CAD build for the part. Positions are in the model's coordinates, mm. A direction names the side the tool comes from. Give positions to 0.01 mm unless a question says otherwise; leave off trailing zeros. Write each loop counter-clockwise with the first axis right and the second up, starting at its lowest first coordinate (ties: lowest second). Pieces come first, ordered by that corner, then holes. Notation, with made-up numbers: (-19.75, 24.5) -> (23.25, 24.5) arc R23 cw to (23.25, 59.5) -> close; hole circle Ø6 at (1.5, -19). An arc over 180 degrees is marked (long way). Answer as a JSON object with one key per item and string values.
Autodesk Inventor part; units mm, degrees
ref_plane "YZ Plane" through (0, 0, 0) normal (1, 0, 0) x (0, 1, 0)
ref_plane "XZ Plane" through (0, 0, 0) normal (0, 1, 0) x (-1, 0, 0)
ref_plane "XY Plane" through (0, 0, 0) normal (0, 0, 1) x (1, 0, 0)
sketch "Sketch1" plane through (0, 0, 0) normal (1, 0, 0) x (0, 1, 0)
  circle A0 centre (4.0001, 0) radius 1.25
  circle A1 centre (-3.9999, 0) radius 1.25
  circle A2 centre (0, 0) radius 11
  line L0 (11, 0) -> (11, -22)
  line L1 (11, 0) -> (33, 0) construction
  line L2 (-11, 0) -> (-11, -22)
  line L3 (-11, 0) -> (11, 0) construction
  circle A3 centre (0, -22) radius 11
  circle A4 centre (0, -26.0001) radius 1.25
  circle A5 centre (0, -18.0001) radius 1.25
  point P0 (1.5875, 1.5875)
  dimension "d0" = 22
  dimension "d1" = 90
  dimension "d2" = 22
  dimension "d3" = 90
extrude "Extrusion1" add sketch "Sketch1" along normal blind 5
sketch "Sketch2" plane through (5, 0, 0) normal (1, 0, 0) x (0, 0, -1)
  arc A0 (0, 11) -> (0, -11) centre (0, 0) ccw
  line L0 (0, -11) -> (22, -11)
  arc A1 (22, -11) -> (22, 11) centre (22, 0) ccw
  line L1 (22, 11) -> (0, 11)
  circle A2 centre (18.0001, 0) radius 1.25
  circle A3 centre (26.0001, 0) radius 1.25
  circle A4 centre (0, -3.9999) radius 1.25
  circle A5 centre (0, 4.0001) radius 1.25
extrude "Extrusion2" add sketch "Sketch2" along normal blind 3 and the other way blind 5 contours A4 | A5
sketch "Sketch3" plane through (0, 0, 0) normal (-1, 0, 0) x (0, 0, 1)
  arc A0 (0, -11) -> (0, 11) centre (0, 0) ccw
  line L0 (0, -11) -> (-22, -11)
  arc A1 (-22, 11) -> (-22, -11) centre (-22, 0) ccw
  line L1 (-22, 11) -> (0, 11)
  circle A2 centre (-18.0001, 0) radius 1.25
  circle A3 centre (-26.0001, 0) radius 1.25
  circle A4 centre (0, -3.9999) radius 1.25
  circle A5 centre (0, 4.0001) radius 1.25
extrude "Extrusion3" add sketch "Sketch3" against normal blind 5 contours A2 | A3
sketch "Sketch4" plane through (0, 0, 0) normal (-1, 0, 0) x (0, 0, 1)
  line L0 (0, 0) -> (-22, 0)
  line L1 (0, 0) -> (22, 0) construction
  circle A0 centre (-22, 0) radius 11
  circle A1 centre (-22, 0) radius 9.5
  dimension "d12" = 22
  dimension "d13" = 180
  dimension "d14" = 22
  dimension "d15" = 19
extrude "Extrusion4" add sketch "Sketch4" along normal blind 15 contours A1 | A0
sketch "Sketch5" plane through (5, 0, 0) normal (1, 0, 0) x (0, 0, -1)
  circle A0 centre (0, 0) radius 24.5
  circle A1 centre (-20, 0) radius 3.5
  circle A2 centre (-14.1421, 14.1421) radius 2.675
  circle A3 centre (-14.1421, -14.1421) radius 2.675
  circle A4 centre (14.1421, -14.1421) radius 2.675
  circle A5 centre (14.1421, 14.1421) radius 2.675
  circle A6 centre (0, 0) radius 11
  line L0 (0, -11) -> (22, -11)
  line L1 (22, 11) -> (0, 11)
  point P0 (0, 0)
  point P1 (21.8918, 11)
  point P2 (21.8918, -11)
extrude "Extrusion5" add sketch "Sketch5" along normal blind 5 contours A0 L0 A6 L1 picked at (19.9018, -1.2624)
sketch "Sketch6" plane through (-15, 0, -22) normal (-1, 0, 0) x (0, 0, 1)
  circle A0 centre (0, 0) radius 7.5
  point P0 (22, 0)
  dimension "d20" = 15
extrude "Extrusion6" cut sketch "Sketch6" against normal blind 15
properties part number "Herramienta Marcador Conector"
1) Mould opens along Y. For faces 1 (the cylindrical face through (-5, 0, -33)), 2 (the flat face through (8, 4, 0)), 3 (the cylindrical face through (6.48, 2.76, 0.16)), 4 (the flat face through (5, 11, -11)) say: released by +Y, released by -Y, zero draft, split by the parting line, or undercut.
Model answer:
{"face 1": "split by the parting line", "face 2": "undercut", "face 3": "undercut", "face 4": "released by +Y"}
2) Slice it at C-C (y = -9). List the corners of the cut face in (x, z), then the cut area to 3 significant figures.
Model answer:
{"outline": "(-15, -28.32) -> (5, -28.32) -> (5, -22.79) -> (10, -22.79) -> (10, -6.32) -> (5, -6.32) -> (5, 6.32) -> (0, 6.32) -> (0, -15.68) -> (-15, -15.68) -> close", "area": "445 mm2"}
3) 3-axis set-ups, long thin cutter, end or side, ignore diameter. For faces 5 (the cylindrical face through (-7.605, 0.33, -29.493)), 6 (the flat face through (8, -4, 0)), 7 (the cylindrical face through (7, 0, -11)), 8 (the cylindrical face through (7.5, 0.2, -24.5)): which of +Z, -Z, +X, -X, +Y, -Y reach the whole face in a straight line?
Model answer:
{"face 5": "-X", "face 6": "+Z, +X", "face 7": "+X", "face 8": "-Z, +X"}
4) Slice it at D-D (x = -9). List the corners of the cut face in (y, z), then the cut area to 3 significant figures.
Model answer:
{"outline": "circle Ø22 at (0, -22); hole circle Ø15 at (0, -22)", "area": "203 mm2"}
5) Pin check, flat tips, straight feed: pin 1 (3 mm diameter, centred on y = -4, z = -0.5, fed in from +X); pin 2 (4.5 mm diameter, centred on y = 3, z = -23, fed in from -X); pin 3 (6 mm diameter, centred on x = 2, y = 8.5, fed in from +Z). Stop position of each tip, or through.
Model answer:
{"pin 1": "stops at x = 8", "pin 2": "stops at x = 0", "pin 3": "stops at z = 9.53"}
6) Slice it at A-A (z = -5.5). List the corners of the cut face in (x, y), then the cut area to 3 significant figures.
Model answer:
{"outline": "(0, -11) -> (10, -11) -> (10, -9.53) -> (5, -9.53) -> (5, 9.53) -> (10, 9.53) -> (10, 11) -> (0, 11) -> close", "area": "125 mm2"}
7) Slice it at B-B (x = 0.75). List the corners of the cut face in (y, z).
Model answer:
{"outline": "(-11, -22) arc R11 ccw to (11, -22) -> (11, 0) arc R11 ccw to (-11, 0) -> close"}
8) Wall check: probe 1 along Y at (x, z) = (-7.5, -22); probe 2 along X at (y, z) = (8, -25); probe 3 along X at (y, z) = (-9.75, -8). Give the ranges that are in metal, low to high.
Model answer:
{"probe 1": "y = -11 to -7.5, 7.5 to 11", "probe 2": "x = -15 to 5", "probe 3": "x = 0 to 10"}
